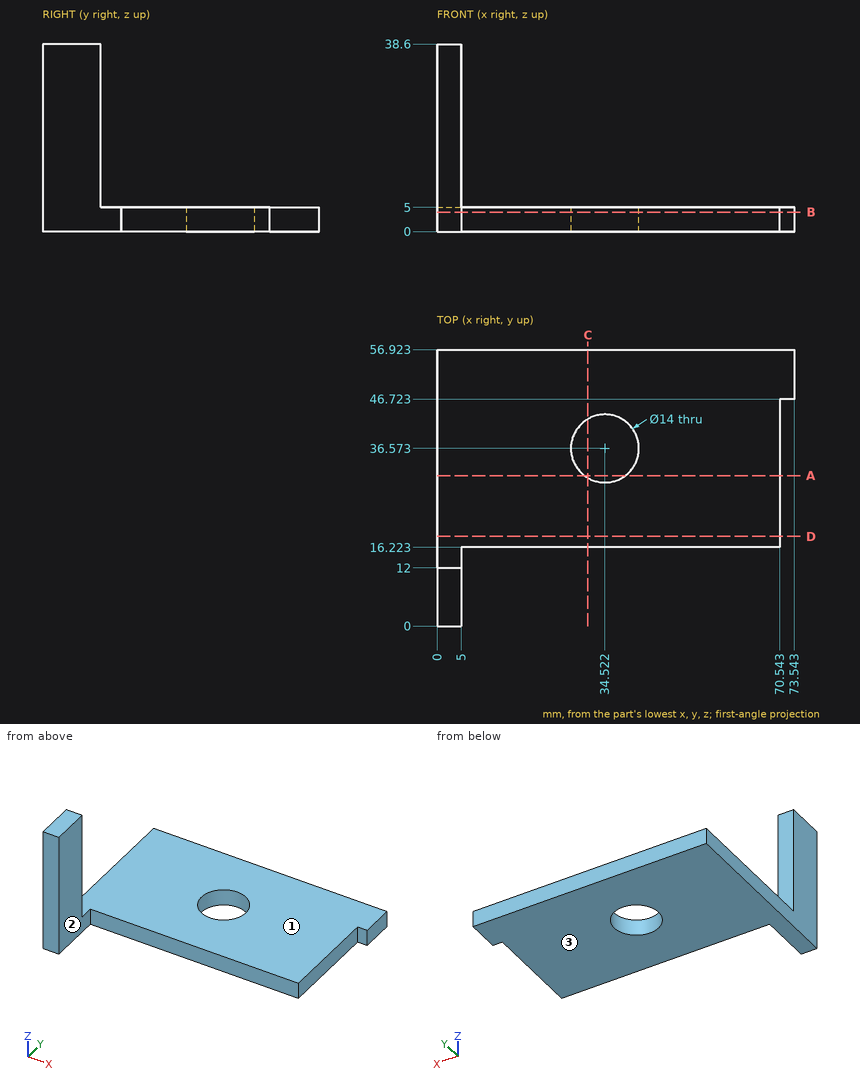
Design review of the part shown in the three views and the two pictorial views. Dimensions are in mm from the part's minimum x, y and z. A direction names the side the tool comes from. Give positions to 0.01 mm unless a question says otherwise; leave off trailing zeros. Write each loop counter-clockwise with the first axis right and the second up, starting at its lowest first coordinate (ties: lowest second). Pieces come first, ordered by that corner, then holes.
Item 1: Wall thickness on probe 1 along Y at (x, z) = (46.5, 2); probe 2 along Y at (x, z) = (29, 4.5) (1 decimal); probe 3 along Z at (x, y) = (52, 44.5): over which ranges is each line inside the solid? List them lowest first.
Item 2: Take a section at A-A (y = 31). Give the boundary of the cut face in (x, z) (1 decimal).
Item 3: Machinability: for the marked faces 1, 2 and 3, which of the approach directions +Z, -Z, +X, -X, +Y, -Y give a long, thin tool a straight path to every point of the face, cutting with its end or side? Answer none if there is none.
Item 4: Take a section at D-D (y = 18.5). Give the boundary of the cut face in (x, z), and give its area (3 significant figures).
Item 5: Take a section at B-B (z = 4). Give the boundary of the cut face in (x, y).
Item 6: Insertion check: P1, Ø6, axis at y = 12.5, z = 20.5, coming from the +X side; P2, Ø10, axis at y = 36, z = 7, coming from the +X side; P3, Ø1, axis at x = 18, y = 19, coming from the +Z side. Each pin has a flat end and moves straight along its axis. Give the tip position at first contact, or say it passes through.
Item 7: Take a section at C-C (x = 31). Give the boundary of the cut face in (y, z).
Established:
1. probe 1: y = 16.22 to 56.92
1. probe 2: y = 16.2 to 32.3, 40.9 to 56.9
1. probe 3: z = 0 to 5
2. outline: (0, 0) - (30.3, 0) - (30.3, 5) - (0, 5) - close; (38.8, 0) - (70.5, 0) - (70.5, 5) - (38.8, 5) - close
3. face 1: +Z, +X, -X, +Y
3. face 2: +Z, -Z, +X, -Y
3. face 3: -Z, +X, -X, +Y, -Y
4. outline: (0, 0) - (70.54, 0) - (70.54, 5) - (0, 5) - close
4. area: 353 mm2
5. outline: (0, 0) - (5, 0) - (5, 16.22) - (70.54, 16.22) - (70.54, 46.72) - (73.54, 46.72) - (73.54, 56.92) - (0, 56.92) - close; hole circle Ø14 at (34.52, 36.57)
6. P1: stops at x = 5
6. P2: stops at x = 70.54
6. P3: stops at z = 5
7. outline: (16.22, 0) - (30.52, 0) - (30.52, 5) - (16.22, 5) - close; (42.62, 0) - (56.92, 0) - (56.92, 5) - (42.62, 5) - close
